```python
from build123d import *

# Parameters (mm, degrees)
PAD005_DEPTH         = 3
SKETCH058_R          = 1.7
POCKET029_DEPTH      = 0.001
POCKET029_DEPTH_BACK = 3.001


with BuildPart() as part:
    # Sketch057 → Pad005 (new body)
    with BuildSketch(Plane.XY):
        with BuildLine():
            ThreePointArc((269.904723, 175.912153), (153.492654, 283.255451), (0, 322.170212))
            Line((0, 322.170212), (0, 342.170212))
            ThreePointArc((287.134265, 186.103111), (163.403661, 300.632163), (0, 342.170212))
            ThreePointArc((286.455952, 183.283279), (287.400483, 184.547572), (287.134265, 186.103111))
            Line((272.580264, 175.272147), (286.455952, 183.283279))
            ThreePointArc((269.904723, 175.912153), (271.114979, 175.059074), (272.580264, 175.272147))
        make_face()
    pad005 = extrude(amount=PAD005_DEPTH)

    # Mirrored011: Pad005 across Sketch057 V_Axis
    add(pad005.mirror(Plane(origin=(0, 0, 0), x_dir=(0, 0, 1), z_dir=(1, 0, 0))))

    # Sketch058 → Pocket029 (cut, two sides)
    with BuildSketch(Plane.XY) as pocket029_sk:
        with Locations((105.577257, 314.945221)):
            Circle(SKETCH058_R)
        with Locations((274.068932, 187.678635)):
            Circle(SKETCH058_R)
        with Locations((-105.577257, 314.945221)):
            Circle(SKETCH058_R)
        with Locations((-274.068932, 187.678635)):
            Circle(SKETCH058_R)
    extrude(amount=-POCKET029_DEPTH, mode=Mode.SUBTRACT)
    extrude(pocket029_sk.sketch, amount=POCKET029_DEPTH_BACK, mode=Mode.SUBTRACT)


solid = part.part
```
Work out the finished part from the listing and answer in its coordinate system (mm). Give positions to 0.01 mm unless a question says otherwise; leave off trailing zeros. Write each loop counter-clockwise with the first axis right and the second up, starting at its lowest first coordinate (ties: lowest second). Pieces come first, ordered by that corner, then holes.
(1) The part is cut by section D-D on x = -60.5. Write down the section's boundary in (y, z), plus the area to 3 significant figures.
Final values:
outline: (316.44, 0) - (336.78, 0) - (336.78, 3) - (316.44, 3) - close
area: 61.0 mm2
(2) A flat-ended cylindrical pin translates along its axis: pin 1 Ø1.5 at (y, z) = (315, 1.5) entering from +X. Find the tip coordinate at first contact, or state that the pin passes through.
Final values:
pin 1: stops at x = 135.38
(3) Straight lines are drawn through the part: line 1 (X direction, y = 206, z = 2.35); line 2 (X direction, y = 294, z = 1.7); line 3 (Y direction, x = 145, z = 2.8). For each, find the intervals that lie inside material, in ascending order.
Final values:
line 1: x = -273.21 to -247.7, 247.7 to 273.21
line 2: x = -175.06 to -131.75, 131.75 to 175.06
line 3: y = 287.7 to 309.93
(4) The part is cut by section B-B on z = 1.15. Write down the section's boundary in (x, y).
Final values:
outline: (-287.13, 186.1) arc R2 ccw to (-286.46, 183.28) - (-272.58, 175.27) arc R2 ccw to (-269.9, 175.91) arc R322.17 cw to (269.9, 175.91) arc R2 ccw to (272.58, 175.27) - (286.46, 183.28) arc R2 ccw to (287.13, 186.1) arc R342.17 ccw to (0, 342.17) arc R342.17 ccw to start; hole circle Ø3.4 at (-274.07, 187.68); hole circle Ø3.4 at (-105.58, 314.95); hole circle Ø3.4 at (105.58, 314.95); hole circle Ø3.4 at (274.07, 187.68)
(5) The part is cut by section C-C on y = 196. Write down the section's boundary in (x, z), plus the area to 3 significant figures.
Final values:
outline: (-280.47, 0) - (-255.69, 0) - (-255.69, 3) - (-280.47, 3) - close; (255.69, 0) - (280.47, 0) - (280.47, 3) - (255.69, 3) - close
area: 149 mm2
(6) The part is cut by section A-A on y = 229. Write down the section's boundary in (x, z).
Final values:
outline: (-254.24, 0) - (-226.61, 0) - (-226.61, 3) - (-254.24, 3) - close; (226.61, 0) - (254.24, 0) - (254.24, 3) - (226.61, 3) - close
